```python
from build123d import *

# Parameters (mm, degrees)
F0_W           = 12.5
F0_H           = 25.4
F1_DEPTH       = 4
F3_D           = 4
F3_CSINK_D     = 7.5
F3_CSINK_ANGLE = 90


with BuildPart() as f1:
    # F0 (on Front) → F1 (new body)
    with BuildSketch(Plane.XZ):
        with Locations((0.696272, 9.18723)):
            Rectangle(F0_W, F0_H)
    extrude(amount=-F1_DEPTH)

    # F3 (through all)
    with Locations(Plane(origin=(0, 4, 0), x_dir=(-1, 0, 0), z_dir=(0, 1, 0))):
        with Locations((-0.696272, 15.88723), (-0.696272, 2.48723)):
            CounterSinkHole(F3_D / 2, F3_CSINK_D / 2, counter_sink_angle=F3_CSINK_ANGLE)


solid = f1.part
```
Source: CAD feature listing. Evaluate the final solid. Frame: model axes, mm. Round coordinates to 2 decimals unless told otherwise and drop trailing zeros. Loops run counter-clockwise (first coordinate to the right, second up) from the corner with the lowest first, then second, coordinate; pieces in that order, holes last.
1. Contact query for a flat-ended pin moving along its axis: pin 1 (4.5 mm diameter, centred on x = 0.7, z = 2.49, fed in from -Y). Output: stop coordinate, or through.
2. Mould query, pull axis Z, two halves, no side actions, for faces 1 (the flat face through (1, 4, 9)), 2 (the flat face through (1, 2, 21.887)), 3 (the cylindrical face through (0.263, 1.109, 13.935)). Classes: released by +Z, released by -Z, zero draft, split by the parting line, or undercut.
3. Section query C-C on y = 2.95. Output: boundary loops of the cut face in (x, z).
4. Section query A-A on y = 0.5. Output: boundary loops of the cut face in (x, z), and give its area (3 significant figures).
5. Section query B-B on x = 1. Give the number of separate pieces and of enclosed holes in the cut face, and give its area (3 significant figures).
6. Ray query, L1, parallel to Z at x = 2, y = 1.05; L2, parallel to Z at x = 2.25, y = 2.2; L3, parallel to X at y = 1.5, z = 4.25. Return the intervals inside material, ascending.
Answers below:
1. pin 1: stops at y = 0
2. face 1: zero draft
2. face 2: released by +Z
2. face 3: undercut
3. outline: (-5.55, -3.51) - (6.95, -3.51) - (6.95, 21.89) - (-5.55, 21.89) - close; hole circle Ø5.4 at (0.7, 2.49); hole circle Ø5.4 at (0.7, 15.89)
4. outline: (-5.55, -3.51) - (6.95, -3.51) - (6.95, 21.89) - (-5.55, 21.89) - close; hole circle Ø4 at (0.7, 2.49); hole circle Ø4 at (0.7, 15.89)
4. area: 292 mm2
5. separate pieces: 3
5. enclosed holes: 0
5. area: 63.8 mm2
6. L1: z = -3.51 to 0.97, 4 to 14.37, 17.4 to 21.89
6. L2: z = -3.51 to 1.23, 3.75 to 14.63, 17.15 to 21.89
6. L3: x = -5.55 to -0.25, 1.64 to 6.95
